Could you check a few things on this model? Use its own coordinates, in mm. A direction names the side the tool comes from. Round coordinates to 2 decimals unless told otherwise and drop trailing zeros. Loops run counter-clockwise (first coordinate to the right, second up) from the corner with the lowest first, then second, coordinate; pieces in that order, holes last. Notation, with made-up numbers: (24.25, 9) -> (30.25, 9) arc R32 cw to (30.25, 37) -> close; hole circle Ø3 at (43, 66.25). An arc over 180 degrees is marked (long way). One line per item, written item: value.
```python
from build123d import *

# Parameters (mm, degrees)
SKETCH_R        = 2.25
PAD_DEPTH       = 23
POCKET_DEPTH    = 19
SKETCH002_R     = 4.05
SKETCH002_R_2   = 2.25
POCKET001_DEPTH = 20.001
SKETCH003_R     = 2.25
POCKET002_DEPTH = 10
SKETCH004_R     = 3.75
POCKET003_DEPTH = 10
SKETCH005_R     = 3.75
POCKET004_DEPTH = 10


with BuildPart() as pocket004:
    # Sketch → Pad (new body)
    with BuildSketch(Plane.XY):
        Polygon((0, -20), (40, -20), (40, 20), (-20, 20), (-20, 0), (0, 0), align=None)
        with Locations((18, 8)):
            Circle(SKETCH_R, mode=Mode.SUBTRACT)
        with Locations((13, -10)):
            Circle(SKETCH_R, mode=Mode.SUBTRACT)
        with Locations((28, -10)):
            Circle(SKETCH_R, mode=Mode.SUBTRACT)
    extrude(amount=PAD_DEPTH)

    # Sketch001 → Pocket (cut)
    with BuildSketch(Plane.XY.offset(23)):
        with BuildLine():
            Line((46, 10), (29, 10))
            ThreePointArc((29, 10), (25.778159, 17.77819), (17.999956, 21))
            Line((17.999956, 21), (0, 21))
            Line((0, 21), (0, -23))
            Line((0, -23), (46, -23))
            Line((46, -23), (46, -12))
            Line((28.629923, -14.455693), (46, -12))
            ThreePointArc((28.629923, -5.544307), (23.5, -10), (28.629923, -14.455693))
            Line((28.629923, -5.544307), (46, -8))
            Line((46, -8), (46, 10))
        make_face()
    extrude(amount=-POCKET_DEPTH, mode=Mode.SUBTRACT)

    # Sketch002 → Pocket001 (cut, through all)
    with BuildSketch(Plane.XZ):
        with Locations((-7, 16)):
            Circle(SKETCH002_R)
        with Locations((-10, 6)):
            Circle(SKETCH002_R_2)
    extrude(amount=-POCKET001_DEPTH, mode=Mode.SUBTRACT)

    # Sketch003 → Pocket002 (cut)
    with BuildSketch(Plane.XY.offset(23)):
        with Locations((35, 15)):
            Circle(SKETCH003_R)
    extrude(amount=-POCKET002_DEPTH, mode=Mode.SUBTRACT)

    # Sketch004 → Pocket003 (cut)
    with BuildSketch(Plane(origin=(0, 20, 0), x_dir=(-1, 0, 0), z_dir=(0, 1, 0))):
        with Locations((10, 6)):
            Circle(SKETCH004_R)
    extrude(amount=-POCKET003_DEPTH, mode=Mode.SUBTRACT)

    # Sketch005 → Pocket004 (cut)
    with BuildSketch(Plane(origin=(0, 0, 0), x_dir=(1, 0, 0), z_dir=(0, 0, -1))):
        with Locations((28, 10)):
            Circle(SKETCH005_R)
    extrude(amount=-POCKET004_DEPTH, mode=Mode.SUBTRACT)


with BuildPart() as part_mirroring:
    # Part__Mirroring: instance of Pocket004
    add(pocket004.part.mirror(Plane(origin=(0, 0, 0), x_dir=(0, -1, 0), z_dir=(1, 0, 0))))


solid = part_mirroring.part
```
(1) Please list where these lines run through material, in increasing order: L1, parallel to X at y = -10, z = 1.3; L2, parallel to Y at x = -18, z = 3.25; L3, parallel to Z at x = 10.5, y = 8.
Results below:
L1: x = -40 to -31.75, -24.25 to -15.25, -10.75 to 0
L2: y = -20 to 5.75, 10.25 to 20
L3: z = 0 to 3.81, 8.19 to 13.96, 18.04 to 23
(2) Imagine slicing it at B-B on z = 16. Write out the boundary of the cut face in (x, y).
Results below:
outline: (-40, -12.85) -> (-28.63, -14.46) arc R4.5 ccw (long way) to (-28.63, -5.54) -> (-40, -7.15) -> close; (-40, 10) -> (-29, 10) arc R11 cw to (-22.58, 20) -> (-40, 20) -> close; (0, 0) -> (2.95, 0) -> (2.95, 20) -> (0, 20) -> close; (11.05, 0) -> (20, 0) -> (20, 20) -> (11.05, 20) -> close; hole circle Ø4.5 at (-35, 15); hole circle Ø4.5 at (-28, -10)
(3) Imagine slicing it at C-C on y = -10. Write out the boundary of the cut face in (x, z), then the cut area to 3 significant figures.
Results below:
outline: (-40, 0) -> (-31.75, 0) -> (-31.75, 10) -> (-30.25, 10) -> (-30.25, 23) -> (-40, 23) -> close; (-25.75, 10) -> (-24.25, 10) -> (-24.25, 0) -> (-15.25, 0) -> (-15.25, 4) -> (-23.5, 4) -> (-23.5, 23) -> (-25.75, 23) -> close; (-10.75, 0) -> (0, 0) -> (0, 4) -> (-10.75, 4) -> close
area: 322 mm²
(4) We'd pull the mould along X, two halves only. Please class faces 5 (the face through (0, -10, 2)), 6 (the face through (-10, 5, 0)), 7 (the face through (-36.038, 13.004, 18.07)): +X half, -X half, draft (parallel to the pull), parting line (faces both ways), or undercut.
Results below:
face 5: +X half
face 6: draft
face 7: undercut
(5) Imagine slicing it at A-A on y = 8. Write out the boundary of the cut face in (x, z), then the cut area to 3 significant figures.
Results below:
outline: (-40, 0) -> (-20.25, 0) -> (-20.25, 4) -> (-40, 4) -> close; (-15.75, 0) -> (20, 0) -> (20, 23) -> (0, 23) -> (0, 4) -> (-15.75, 4) -> close; hole circle Ø8.1 at (7, 16); hole circle Ø4.5 at (10, 6)
area: 535 mm²
(6) Imagine slicing it at D-D on x = 7. Write out the boundary of the cut face in (y, z).
Results below:
outline: (0, 0) -> (20, 0) -> (20, 3.75) -> (10, 3.75) -> (10, 8.25) -> (20, 8.25) -> (20, 11.95) -> (0, 11.95) -> close; (0, 20.05) -> (20, 20.05) -> (20, 23) -> (0, 23) -> close
(7) For pin 1 Ø6 at (y, z) = (-1.5, 16) entering from -X; pin 2 Ø20 at (x, y) = (-12, 5) entering from +Z; pin 3 Ø5.5 at (x, z) = (-34.5, 12.5) entering from -Y, each with a flat end and sliding along its axis, tell me the tip position at first contact or that it passes through.
Results below:
pin 1: stops at x = 0
pin 2: stops at z = 4
pin 3: stops at y = -14.01
(8) On a 3-axis mill with a long thin cutter (end or side, diameter ignored), from which of +Z, -Z, +X, -X, +Y, -Y can I reach the whole of each face in a straight line? I mean faces 1 (the face through (-30, -8, 10)), 2 (the face through (10, 0, 11)), 3 (the face through (-34.235, -6.337, 13.633)), 4 (the face through (7.024, 15.07, 3.718)). Say none if no direction works.
Results below:
face 1: -Z
face 2: +Z, -Z, +X, -Y
face 3: +Z, -X
face 4: +Y
